Can you work these out from the model? Positions are in its coordinate system, mm. Face numbers are marked on the shaded views. A direction names the side the tool comes from. Round coordinates to 2 decimals unless told otherwise and drop trailing zeros. Loops run counter-clockwise (first coordinate to the right, second up) from the corner with the lowest first, then second, coordinate; pieces in that order, holes last. Notation, with made-up numbers: (-39.75, 25) -> (0.25, 25) arc R37 cw to (0.25, 62) -> close; hole circle Ø1 at (-21, 2). An arc over 180 degrees is marked (long way). Write item = value, one per line.
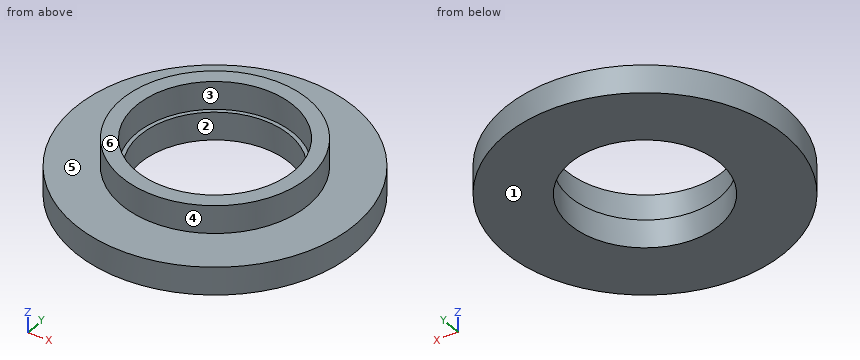
Autodesk Inventor part; units mm, degrees
ref_plane "YZ Plane" through (0, 0, 0) normal (1, 0, 0) x (0, 1, 0)
ref_plane "XZ Plane" through (0, 0, 0) normal (0, 1, 0) x (-1, 0, 0)
ref_plane "XY Plane" through (0, 0, 0) normal (0, 0, 1) x (1, 0, 0)
sketch "Sketch1" plane through (0, 0, 0) normal (0, 0, 1) x (1, 0, 0)
  circle A0 centre (0, 0) radius 8
  circle A1 centre (0, 0) radius 15
  dimension "d0" = 16
  dimension "d1" = 30
extrude "Extrusion1" add sketch "Sketch1" along normal blind 3
sketch "Sketch2" plane through (0, 0, 3) normal (0, 0, 1) x (1, 0, 0)
  circle A0 centre (0, 0) radius 8.4211
  circle A1 centre (0, 0) radius 10
  dimension "d4" = 20
extrude "Extrusion2" add sketch "Sketch2" along normal blind 3
properties part number "bushing"
1. I'm going to push flat-ended pins straight in: pin 1 (3 mm diameter, centred on y = 8.5, z = 5, fed in from +X); pin 2 (3 mm diameter, centred on x = -10, z = 2, fed in from -Y); pin 3 (1.5 mm diameter, centred on x = -3.5, z = 3, fed in from -Y). Where does each tip first touch, or does it pass through?
Entries:
pin_1 = 7.14
pin_2 = -12.36
pin_3 = -14.75
2. I need wall thicknesses on line 1 (Y direction, x = 0, z = 1.5); line 2 (Y direction, x = 0, z = 3.95); line 3 (Z direction, x = 8.25, y = 0). Which ranges of each line are inside material? Lowest first, please. Write a range as [from, to].
Entries:
line_1 = [-15, -8], [8, 15]
line_2 = [-10, -8.42], [8.42, 10]
line_3 = [0, 3]
3. We'd pull the mould along Y, two halves only. Please class the marked faces 1, 2, 3 and 4: released by +Y, released by -Y, zero draft, split by the parting line, or undercut.
Entries:
face_1 = zero draft
face_2 = undercut
face_3 = undercut
face_4 = split by the parting line
4. For the marked faces 5 and 6, which set-ups out of +Z, -Z, +X, -X, +Y, -Y let a thin tool reach every point of the face, with its end or its side?
Entries:
face_5 = +Z
face_6 = +Z, +X, -X, +Y, -Y
5. Suppose I cut it at A-A, the plane x = 0. List the corners of the cut face in (y, z) for me.
Entries:
outline = (-15, 0) -> (-8, 0) -> (-8, 3) -> (-8.42, 3) -> (-8.42, 6) -> (-10, 6) -> (-10, 3) -> (-15, 3) -> close; (8, 0) -> (15, 0) -> (15, 3) -> (10, 3) -> (10, 6) -> (8.42, 6) -> (8.42, 3) -> (8, 3) -> close
6. Suppose I cut it at D-D, the plane y = 9. List the corners of the cut face in (x, z) for me.
Entries:
outline = (-12, 0) -> (12, 0) -> (12, 3) -> (4.36, 3) -> (4.36, 6) -> (-4.36, 6) -> (-4.36, 3) -> (-12, 3) -> close
7. Suppose I cut it at B-B, the plane y = 3.75. List the corners of the cut face in (x, z) for me, and give its area (3 significant figures).
Entries:
outline = (-14.52, 0) -> (-7.07, 0) -> (-7.07, 3) -> (-7.54, 3) -> (-7.54, 6) -> (-9.27, 6) -> (-9.27, 3) -> (-14.52, 3) -> close; (7.07, 0) -> (14.52, 0) -> (14.52, 3) -> (9.27, 3) -> (9.27, 6) -> (7.54, 6) -> (7.54, 3) -> (7.07, 3) -> close
area = 55.1 mm²
8. Suppose I cut it at C-C, the plane z = 1.35. List the corners of the cut face in (x, y) for me, and give its area (3 significant figures).
Entries:
outline = circle Ø30 at (0, 0); hole circle Ø16 at (0, 0)
area = 506 mm²
